Job drawing, mm, ordinate dimensions from the low corner. One solid piece. A direction names the side the tool comes from. Coordinates: 2 decimals unless noted, no trailing zeros. Loops run counter-clockwise (first coordinate to the right, second up) from the corner with the lowest first, then second, coordinate; pieces in that order, holes last. Notation, with made-up numbers: (49, 45) -> (84, 45) arc R21 ccw to (84, 67) -> close; hole circle Ø6 at (-9, -26). An arc over 180 degrees is marked (long way). Answer as CSV lines item,"result". Start each with the question number.
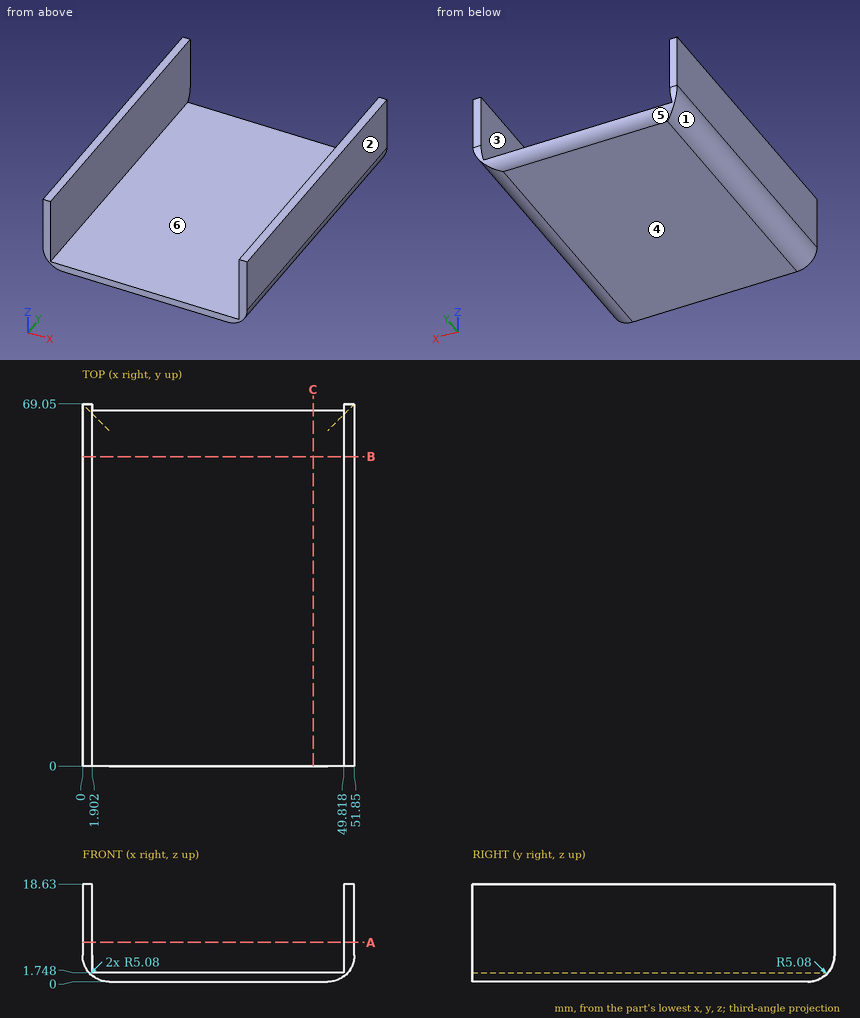
Item 1: Which spindle directions (+Z, -Z, +X, -X, +Y, -Y) get a long thin tool onto all of the face, cutting with end or side? Do the marked faces 5 and 6. Say none if no direction does.
Item 2: Saw through at A-A (z = 7.5). Write the cut outline in (x, y).
Item 3: Saw through at C-C (x = 44). Write the cut outline in (y, z) (1 decimal).
Item 4: Two-plate mould, pull along X, no slides. Class the marked faces 1, 2, 3 and 4: pulls with the +X half, pulls with the -X half, needs draft (parallel to the pull), parting line crosses it, or undercut.
Item 5: Flat gauge pin, fed straight in: pin 1 Ø14.5 at (x, y) = (35, 28) entering from +Z. Where does the tip first touch, or does it go through?
Item 6: Wall check: probe 1 along X at (y, z) = (10.5, 7.75); probe 2 along Z at (x, y) = (9, 38); probe 3 along X at (y, z) = (63.5, 3.5). Give the ranges that are in metal, low to high.
Item 7: Saw through at B-B (y = 59). Write the cut outline in (x, z), plus the area to 3 significant figures.
Geometry check:
1,face 5,"-Z, +X, -X, +Y"
1,face 6,"+Z, +Y, -Y"
2,outline,"(0, 0) -> (1.9, 0) -> (1.9, 69.05) -> (0, 69.05) -> close; (49.82, 0) -> (51.85, 0) -> (51.85, 69.05) -> (49.82, 69.05) -> close"
3,outline,"(0, 0) -> (64, 0) arc R5.1 ccw to (67.8, 1.7) -> (0, 1.7) -> close"
4,face 1,"pulls with the -X half"
4,face 2,"pulls with the +X half"
4,face 3,"undercut"
4,face 4,"needs draft"
5,pin 1,"z = 1.75"
6,probe 1,"0 to 1.9, 49.82 to 51.85"
6,probe 2,"0 to 1.75"
6,probe 3,"0.25 to 1.9, 49.82 to 51.6"
7,outline,"(0, 5.08) arc R5.08 ccw to (5.08, 0) -> (46.77, 0) arc R5.08 ccw to (51.85, 5.08) -> (51.85, 18.63) -> (49.82, 18.63) -> (49.82, 1.75) -> (1.9, 1.75) -> (1.9, 18.63) -> (0, 18.63) -> close"
7,area,"146 mm2"
